Source: CAD feature listing. Evaluate the final solid. Frame: model axes, mm. Give positions to 0.01 mm unless a question says otherwise; leave off trailing zeros. Order: outer loops, then holes, each group sorted by start corner. A loop starts at its lowest first (then second) coordinate and runs counter-clockwise, first axis right, second up. Notation, with made-up numbers: (4.25, 70) - (63.25, 70) arc R22 ccw to (63.25, 80) - close; hole circle Ø10 at (42.25, -30.5). An arc over 180 degrees is marked (long way). One line per item, written item: value. Start each with the question number.
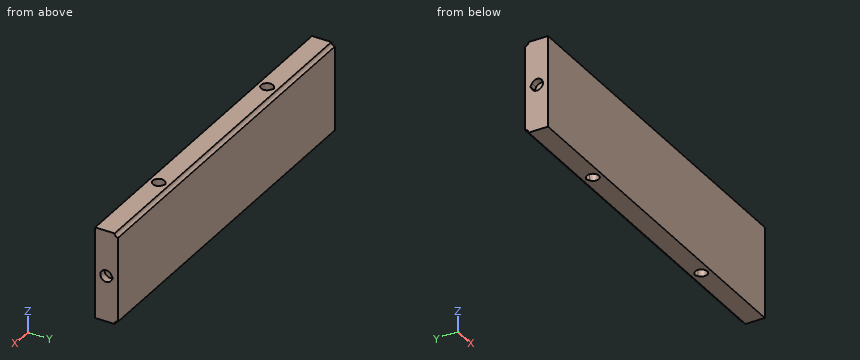
from build123d import *

# Parameters (mm, degrees)
SKETCH_1_W                         = 160
SKETCH_1_H                         = 40
EXTRUDE_1_DEPTH                    = 10
SWEEP_START                        = -80
SWEEP_1_DEPTH                      = 160
SWEEP_2_DEPTH                      = 160
SKETCH_16_R                        = 2.575
CUT_EXTRUDE_1_DEPTH                = 3.15
PATTERN_LINEAR_1_COUNT             = 2
PATTERN_LINEAR_1_PITCH             = 80
PATTERN_CIRCULAR_1_COUNT           = 2
PATTERN_CIRCULAR_1_COPY_1_SKETCH_R = 2.575
PATTERN_CIRCULAR_1_COPY_1_DEPTH    = 3.15
SKETCH_20_R                        = 2.575
CUT_EXTRUDE_2_DEPTH                = 3.15
PATTERN_CIRCULAR_2_COUNT           = 2


# Read off the part's stored shape, not the designer's step: Вырез-По траектории1, Вырез-По траектории2
with BuildPart() as part:
    # Эскиз1 → Бобышка-Вытянуть1 (new body)
    with BuildSketch(Plane(origin=(0, 0, 0), x_dir=(1, 0, 0), z_dir=(0, 1, 0))):
        Rectangle(SKETCH_1_W, SKETCH_1_H)
    extrude(amount=-EXTRUDE_1_DEPTH)

    # Вырез-По траектории1 outline → Вырез-По траектории1 (cut)
    with BuildSketch(Plane.YZ.offset(SWEEP_START)):
        with BuildLine():
            Line((0, 20), (-1.5, 20))
            ThreePointArc((-1.5, 20), (-1.060660172, 18.939339828), (0, 18.5))
            Line((0, 18.5), (0, 20))
        make_face()
    extrude(amount=SWEEP_1_DEPTH, mode=Mode.SUBTRACT)

    # Вырез-По траектории2 outline → Вырез-По траектории2 (cut)
    with BuildSketch(Plane.YZ.offset(SWEEP_START)):
        with BuildLine():
            ThreePointArc((0, -18.5), (-1.060660172, -18.939339828), (-1.5, -20))
            Line((-1.5, -20), (0, -20))
            Line((0, -20), (0, -18.5))
        make_face()
    extrude(amount=SWEEP_2_DEPTH, mode=Mode.SUBTRACT)

    # Эскиз16 → Вырез-Вытянуть1 (cut)
    with BuildSketch(Plane(origin=(0, 0, -20), x_dir=(-1, 0, 0), z_dir=(0, 0, -1))):
        with Locations((-40, -5.949176943)):
            Circle(SKETCH_16_R)
        with BuildLine():
            Line((-40, -2.975823057), (-41.2875, -3.719161528))
            ThreePointArc((-41.2875, -3.719161528), (-40, -3.374176943), (-38.7125, -3.719161528))
            Line((-38.7125, -3.719161528), (-40, -2.975823057))
        make_face()
    cut_extrude_1 = extrude(amount=-CUT_EXTRUDE_1_DEPTH, mode=Mode.SUBTRACT)

    # Линейный массив1: Вырез-Вытянуть1 ×2
    with Locations(*[(-i * PATTERN_LINEAR_1_PITCH, 0, 0) for i in range(1, PATTERN_LINEAR_1_COUNT)]):
        add(cut_extrude_1, mode=Mode.SUBTRACT)

    # Круговой массив1: Вырез-Вытянуть1 ×2 about axis
    pattern_circular_1_axis = Axis((0, -10, 0), (0, -1, 0))
    for i in range(1, PATTERN_CIRCULAR_1_COUNT):
        add(cut_extrude_1.rotate(pattern_circular_1_axis, i * 360 / PATTERN_CIRCULAR_1_COUNT), mode=Mode.SUBTRACT)

    # Круговой массив1 copy 1 sketch → Круговой массив1 copy 1 (cut)
    with BuildSketch(Plane(origin=(80, 0, 20), x_dir=(1, 0, 0), z_dir=(0, 0, 1))):
        with Locations((-40, -5.949176943)):
            Circle(PATTERN_CIRCULAR_1_COPY_1_SKETCH_R)
        with BuildLine():
            Line((-40, -2.975823057), (-41.2875, -3.719161528))
            ThreePointArc((-41.2875, -3.719161528), (-40, -3.374176943), (-38.7125, -3.719161528))
            Line((-38.7125, -3.719161528), (-40, -2.975823057))
        make_face()
    extrude(amount=-PATTERN_CIRCULAR_1_COPY_1_DEPTH, mode=Mode.SUBTRACT)

    # Эскиз20 → Вырез-Вытянуть2 (cut)
    with BuildSketch(Plane.ZY.offset(-80)):
        with Locations((0, -5.199176943)):
            Circle(SKETCH_20_R)
        with BuildLine():
            Line((1.2875, -2.969161528), (0, -2.225823057))
            Line((0, -2.225823057), (-1.2875, -2.969161528))
            ThreePointArc((-1.2875, -2.969161528), (0, -2.624176943), (1.2875, -2.969161528))
        make_face()
    cut_extrude_2 = extrude(amount=CUT_EXTRUDE_2_DEPTH, mode=Mode.SUBTRACT)

    # Круговой массив2: Вырез-Вытянуть2 ×2 about axis
    pattern_circular_2_axis = Axis((0, -10, 0), (0, -1, 0))
    for i in range(1, PATTERN_CIRCULAR_2_COUNT):
        add(cut_extrude_2.rotate(pattern_circular_2_axis, i * 360 / PATTERN_CIRCULAR_2_COUNT), mode=Mode.SUBTRACT)


solid = part.part
1. Ray query, L1, parallel to Y at x = 40, z = -19.2; L2, parallel to Y at x = 40, z = 17.7; L3, parallel to X at y = -3.75, z = -17. Return the intervals inside material, ascending.
2. Contact query for flat-ended pins moving along their axis: pin 1 Ø4 at (y, z) = (-4.5, 1) entering from -X; pin 2 Ø2.5 at (x, y) = (39.5, -5) entering from +Z; pin 3 Ø2.5 at (x, y) = (39, -6.5) entering from -Z; pin 4 Ø4.5 at (y, z) = (-5.2, 0) entering from -X. Output: stop coordinate, or through.
3. Section A-A on y = -5.75. Return the cut outline in (x, z), then the cut area to 3 significant figures.
Data:
1. L1: y = -10 to -8.52, -2.98 to -1.27
1. L2: y = -10 to -8.52, -2.98 to 0
1. L3: x = -80 to -41.34, -38.66 to 38.66, 41.34 to 80
2. pin 1: stops at x = -80
2. pin 2: stops at z = 16.85
2. pin 3: stops at z = -16.85
2. pin 4: stops at x = -76.85
3. outline: (-80, -20) - (-42.57, -20) - (-42.57, -16.85) - (-37.43, -16.85) - (-37.43, -20) - (37.43, -20) - (37.43, -16.85) - (42.57, -16.85) - (42.57, -20) - (80, -20) - (80, -2.52) - (76.85, -2.52) - (76.85, 2.52) - (80, 2.52) - (80, 20) - (42.57, 20) - (42.57, 16.85) - (37.43, 16.85) - (37.43, 20) - (-37.43, 20) - (-37.43, 16.85) - (-42.57, 16.85) - (-42.57, 20) - (-80, 20) - (-80, 2.52) - (-76.85, 2.52) - (-76.85, -2.52) - (-80, -2.52) - close
3. area: 6,300 mm2
